The model under review builds one solid part; all positions refer to its coordinate system, in mm. Round coordinates to 2 decimals unless told otherwise and drop trailing zeros. Write each loop counter-clockwise with the first axis right and the second up, starting at its lowest first coordinate (ties: lowest second). Pieces come first, ordered by that corner, then holes. Notation, with made-up numbers: (-36.75, -16.5) -> (-18.75, -16.5) arc R20 ccw to (-18.75, 10.5) -> close; hole circle Ø1 at (-30.5, -5). An arc over 180 degrees is marked (long way). Answer as a JSON object with one key per item and string values. Group by question number.
1) To check wall thickness, follow probe 1 along Y at (x, z) = (96, 1.05); probe 2 along Y at (x, z) = (92, 1.35); probe 3 along X at (y, z) = (32.5, 1.3). State the ranges of each line that lie inside material, in increasing order. Write a range as [from, to].
2) We need section A-A, the plane y = 63.5. Write out the cut boundary in (x, z), then the cut area to 3 significant figures.
3) We need section B-B, the plane x = 10. Write out the cut boundary in (y, z), then the cut area to 3 significant figures.
4) Insertion check: pin 1 Ø3 at (x, y) = (4, 4) entering from +Z. The pin has a flat end and moves straight along its axis. Give the tip position at first contact, or say it passes through.
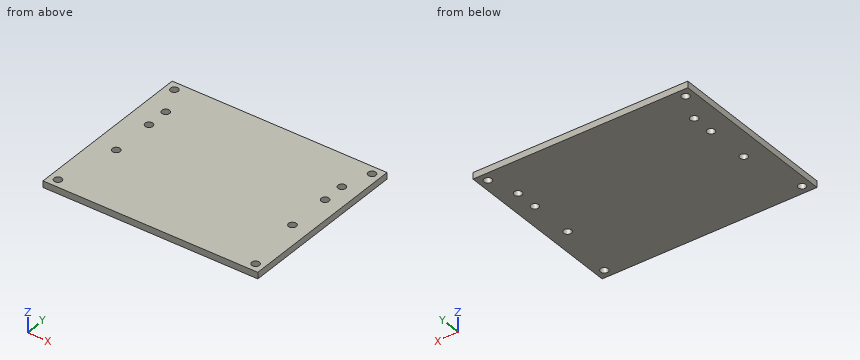
from build123d import *

# Parameters (mm, degrees)
CYLINDER012_R     = 1.8
CYLINDER012_DEPTH = 20
ARRAY007_X_COUNT  = 2
ARRAY007_X_PITCH  = 92
ARRAY007_Y_COUNT  = 2
ARRAY007_Y_PITCH  = 73
CYLINDER013_R     = 1.8
CYLINDER013_DEPTH = 20
ARRAY008_X_COUNT  = 2
ARRAY008_X_PITCH  = 82
CYLINDER011_R     = 1.8
CYLINDER011_DEPTH = 20
ARRAY_X_COUNT     = 2
ARRAY_X_PITCH     = 82
ARRAY_Y_COUNT     = 2
ARRAY_Y_PITCH     = 31
BOX_W             = 100
BOX_H             = 81
BOX_DEPTH         = 3


with BuildPart() as corner_hole_array:
    # Cylinder012 → Cylinder012 (new body)
    with BuildSketch(Plane(origin=(4, 4, -6), x_dir=(1, 0, 0), z_dir=(0, 0, 1))):
        Circle(CYLINDER012_R)
    extrude(amount=CYLINDER012_DEPTH)

    # Array007 X: corner hole array ×2


with BuildPart() as corner_hole_array_1:
    add(corner_hole_array.part)
    with Locations(*[(i * ARRAY007_X_PITCH, 0, 0) for i in range(1, ARRAY007_X_COUNT)]):
        add(corner_hole_array.part)

    # Array007 Y: corner hole array ×2


with BuildPart() as corner_hole_array_2:
    add(corner_hole_array_1.part)
    with Locations(*[(0, i * ARRAY007_Y_PITCH, 0) for i in range(1, ARRAY007_Y_COUNT)]):
        add(corner_hole_array_1.part)


with BuildPart() as screw_hole_array:
    # Cylinder013 → Cylinder013 (new body)
    with BuildSketch(Plane(origin=(10, 53, -6), x_dir=(1, 0, 0), z_dir=(0, 0, 1))):
        Circle(CYLINDER013_R)
    extrude(amount=CYLINDER013_DEPTH)

    # Array008 X: screw hole array ×2


with BuildPart() as screw_hole_array_1:
    add(screw_hole_array.part)
    with Locations(*[(i * ARRAY008_X_PITCH, 0, 0) for i in range(1, ARRAY008_X_COUNT)]):
        add(screw_hole_array.part)


with BuildPart() as hole_fusion:
    # Cylinder011 → Cylinder011 (new body)
    with BuildSketch(Plane(origin=(10, 32.5, -6), x_dir=(1, 0, 0), z_dir=(0, 0, 1))):
        Circle(CYLINDER011_R)
    extrude(amount=CYLINDER011_DEPTH)

    # Array X: hole fusion ×2


with BuildPart() as hole_fusion_1:
    add(hole_fusion.part)
    with Locations(*[(i * ARRAY_X_PITCH, 0, 0) for i in range(1, ARRAY_X_COUNT)]):
        add(hole_fusion.part)

    # Array Y: hole fusion ×2


with BuildPart() as hole_fusion_2:
    add(hole_fusion_1.part)
    with Locations(*[(0, i * ARRAY_Y_PITCH, 0) for i in range(1, ARRAY_Y_COUNT)]):
        add(hole_fusion_1.part)

    # Fusion: union corner hole array, screw hole array
    add(corner_hole_array_2.part)
    add(screw_hole_array_1.part)


with BuildPart() as bottom_part_cut:
    # Box → Box (new body)
    with BuildSketch(Plane.XY):
        with Locations((50, 40.5)):
            Rectangle(BOX_W, BOX_H)
    extrude(amount=BOX_DEPTH)

    # Cut008: cut hole fusion
    add(hole_fusion_2.part, mode=Mode.SUBTRACT)


solid = bottom_part_cut.part
Here are the results:
{
 "1": {"probe 1": "y = [0, 2.2], [5.8, 75.2], [78.8, 81]", "probe 2": "y = [0, 30.7], [34.3, 51.2], [54.8, 61.7], [65.3, 81]", "probe 3": "x = [0, 8.2], [11.8, 90.2], [93.8, 100]"},
 "2": {"outline": "(0, 0) -> (8.2, 0) -> (8.2, 3) -> (0, 3) -> close; (11.8, 0) -> (90.2, 0) -> (90.2, 3) -> (11.8, 3) -> close; (93.8, 0) -> (100, 0) -> (100, 3) -> (93.8, 3) -> close", "area": "278 mm^2"},
 "3": {"outline": "(0, 0) -> (30.7, 0) -> (30.7, 3) -> (0, 3) -> close; (34.3, 0) -> (51.2, 0) -> (51.2, 3) -> (34.3, 3) -> close; (54.8, 0) -> (61.7, 0) -> (61.7, 3) -> (54.8, 3) -> close; (65.3, 0) -> (81, 0) -> (81, 3) -> (65.3, 3) -> close", "area": "211 mm^2"},
 "4": {"pin 1": "passes through"}
}
